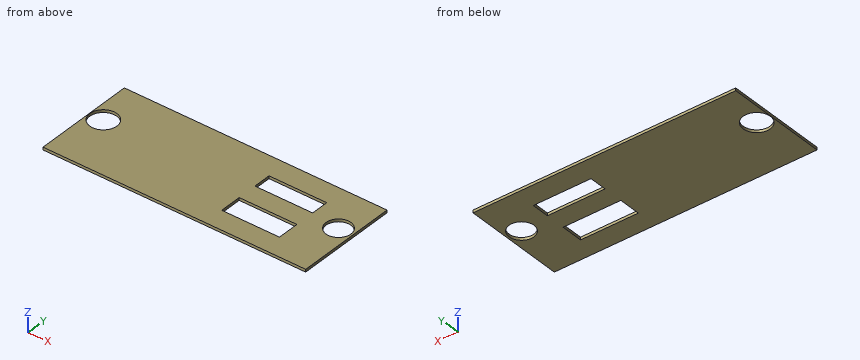
from build123d import *

# Parameters (mm, degrees)
F0_W     = 97.523712
F0_H     = 37.792742
F1_DEPTH = 1
F2_R     = 4.623594
F2_R_2   = 5.035286
F3_DEPTH = 25.4
F4_W     = 21.440587
F4_H     = 8.105589
F5_DEPTH = 25.4


with BuildPart() as f1:
    # F0 (on Top) → F1 (new body)
    with BuildSketch(Plane.XY):
        Rectangle(F0_W, F0_H)
    extrude(amount=F1_DEPTH)

    # F2 (on face) → F3 (cut)
    with BuildSketch(Plane.XY.offset(1)):
        with Locations((43.415565, 3.041855)):
            Circle(F2_R)
        with Locations((-43.599922, 2.673145)):
            Circle(F2_R_2)
    extrude(amount=-F3_DEPTH, mode=Mode.SUBTRACT)

    # F4 (on face) → F5 (cut)
    with BuildSketch(Plane.XY.offset(1)):
        Polygon((32.814559, 4.314265), (32.814559, 10.85103), (11.373972, 10.85103), (11.373972, 4.314265), (13.988677, 4.314265), align=None)
        with Locations((22.094265, -7.059706)):
            Rectangle(F4_W, F4_H)
    extrude(amount=-F5_DEPTH, mode=Mode.SUBTRACT)


solid = f1.part
Geometry: final body of the model. Coordinates: model frame, mm. Give positions to 0.01 mm unless a question says otherwise; leave off trailing zeros. Write each loop counter-clockwise with the first axis right and the second up, starting at its lowest first coordinate (ties: lowest second). Pieces come first, ordered by that corner, then holes.
(1) Cut plane B-B, the plane x = -42.5. Return loops of the section in (y, z), then the cut area to 3 significant figures.
(2) Cut plane D-D, the plane y = 6. Return loops of the section in (x, z).
(3) Cut plane C-C, the plane z = 0.25. Return loops of the section in (x, y), then the cut area to 3 significant figures.
(4) Ray query, line 1 (Y direction, x = 17.5, z = 0.9); line 2 (X direction, y = 10.5, z = 0.8); line 3 (Y direction, x = -43.5, z = 0.65). Return the intervals inside material, ascending.
(5) First-contact query: P1, Ø16, axis at x = -43.6, y = 2.67, coming from the -Z side. Flat tip, straight axial feed; report the tip coordinate or a pass-through.
(6) Cut plane A-A, the plane y = -10. Return loops of the section in (x, z), then the cut area to 3 significant figures.
Values follow:
1. outline: (-18.9, 0) - (-2.24, 0) - (-2.24, 1) - (-18.9, 1) - close; (7.59, 0) - (18.9, 0) - (18.9, 1) - (7.59, 1) - close
1. area: 28.0 mm2
2. outline: (-48.76, 0) - (-47.38, 0) - (-47.38, 1) - (-48.76, 1) - close; (-39.82, 0) - (11.37, 0) - (11.37, 1) - (-39.82, 1) - close; (32.81, 0) - (39.86, 0) - (39.86, 1) - (32.81, 1) - close; (46.97, 0) - (48.76, 0) - (48.76, 1) - (46.97, 1) - close
3. outline: (-48.76, -18.9) - (48.76, -18.9) - (48.76, 18.9) - (-48.76, 18.9) - close; hole circle Ø10.07 at (-43.6, 2.67); hole (11.37, -11.11) - (32.81, -11.11) - (32.81, -3.01) - (11.37, -3.01) - close; hole (11.37, 4.31) - (32.81, 4.31) - (32.81, 10.85) - (11.37, 10.85) - close; hole circle Ø9.25 at (43.42, 3.04)
3. area: 3,220 mm2
4. line 1: y = -18.9 to -11.11, -3.01 to 4.31, 10.85 to 18.9
4. line 2: x = -48.76 to 11.37, 32.81 to 48.76
4. line 3: y = -18.9 to -2.36, 7.71 to 18.9
5. P1: stops at z = 0
6. outline: (-48.76, 0) - (11.37, 0) - (11.37, 1) - (-48.76, 1) - close; (32.81, 0) - (48.76, 0) - (48.76, 1) - (32.81, 1) - close
6. area: 76.1 mm2
